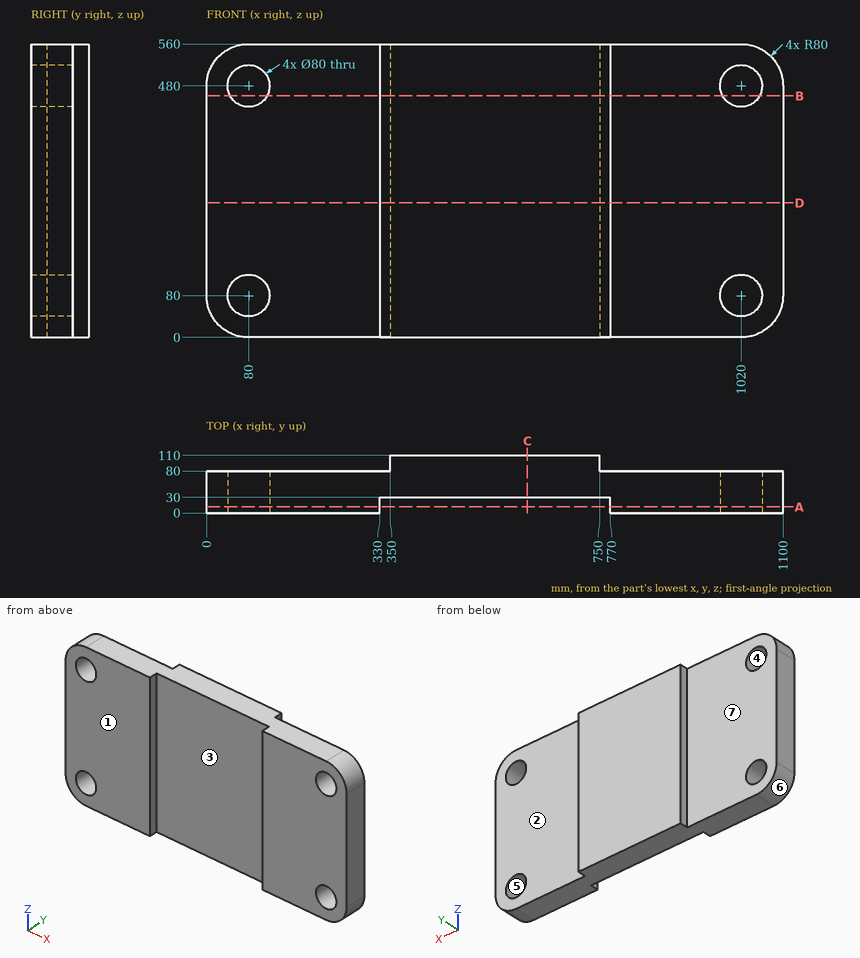
Input: dimensioned drawing with shaded views. Units: mm. Origin: part minimum x, y, z. A direction names the side the tool comes from. Round coordinates to 2 decimals unless told otherwise and drop trailing zeros. Loops run counter-clockwise (first coordinate to the right, second up) from the corner with the lowest first, then second, coordinate; pieces in that order, holes last. Notation, with made-up numbers: M 55,11 L 105,11 A26 ccw 105,38 Z; hole C -28,29.5 d6. An arc over 180 degrees is marked long. Return JSON: item names as keys, results as strings. Group by question number.
1. Material intervals for line 1 along Z through (x, y) = (1018, 68); line 2 along X through (y, z) = (21.5, 380.5); line 3 along X through (y, z) = (45, 455.5), sorted ascending. Write a range as from..to.
2. Mould query, pull axis Z, two halves, no side actions, for the marked faces 4, 5, 6 and 7. Classes: released by +Z, released by -Z, zero draft, split by the parting line, or undercut.
3. Section query B-B on z = 461. Output: boundary loops of the cut face in (x, y).
4. Pin query (flat end, axial travel): pin 1 (9 mm diameter, centred on y = 100, z = 288.5, fed in from -X); pin 2 (1 mm diameter, centred on x = 671.5, z = 210, fed in from -Y); pin 3 (1.5 mm diameter, centred on y = 88.5, z = 83, fed in from +X). Return the tip coordinate at first contact, or that it passes through.
5. Section query A-A on y = 12. Output: boundary loops of the cut face in (x, z).
6. Section query C-C on x = 612. Output: boundary loops of the cut face in (y, z).
7. Reachability of the marked faces 1, 2 and 3 from +Z, -Z, +X, -X, +Y, -Y: full face, straight path, thin tool, end or side. Return the list, or none.
8. Section query D-D on z = 257. Output: boundary loops of the cut face in (x, y), and give its area (3 significant figures).
Checks:
{
 "1": {"line 1": "z = 0..40.05, 119.95..440.05, 519.95..560", "line 2": "x = 0..330, 770..1100", "line 3": "x = 0..48.38, 111.62..988.38, 1051.62..1100"},
 "2": {"face 4": "undercut", "face 5": "undercut", "face 6": "released by -Z", "face 7": "zero draft"},
 "3": {"outline": "M 0,0 L 44.8,0 L 44.8,80 L 0,80 Z; M 115.2,0 L 330,0 L 330,30 L 770,30 L 770,0 L 984.8,0 L 984.8,80 L 750,80 L 750,110 L 350,110 L 350,80 L 115.2,80 Z; M 1055.2,0 L 1100,0 L 1100,80 L 1055.2,80 Z"},
 "4": {"pin 1": "stops at x = 350", "pin 2": "stops at y = 30", "pin 3": "stops at x = 750"},
 "5": {"outline": "M 0,80 A80 ccw 80,0 L 330,0 L 330,560 L 80,560 A80 ccw 0,480 Z; M 770,0 L 1020,0 A80 ccw 1100,80 L 1100,480 A80 ccw 1020,560 L 770,560 Z; hole C 80,80 d80; hole C 80,480 d80; hole C 1020,80 d80; hole C 1020,480 d80"},
 "6": {"outline": "M 30,0 L 110,0 L 110,560 L 30,560 Z"},
 "7": {"face 1": "+Z, -Z, +X, -X, -Y", "face 2": "+Z, -Z, +X, +Y", "face 3": "+Z, -Z, -Y"},
 "8": {"outline": "M 0,0 L 330,0 L 330,30 L 770,30 L 770,0 L 1100,0 L 1100,80 L 750,80 L 750,110 L 350,110 L 350,80 L 0,80 Z", "area": "86,800 mm²"}
}
